```python
from build123d import *

# Parameters (mm, degrees)
SKETCH1_W           = 50
SKETCH1_H           = 200
BOSS_EXTRUDE1_DEPTH = 5.2
SKETCH2_W           = 4.9
SKETCH2_H           = 7.8
SKETCH2_W_2         = 5.7
SKETCH2_H_2         = 9
SKETCH2_W_3         = 25
SKETCH2_H_3         = 4.9
CUT_EXTRUDE1_DEPTH  = 5.2
CHAMFER2_SIZE       = 2.6


with BuildPart() as part:
    # Sketch1 → Boss-Extrude1 (new body)
    with BuildSketch(Plane(origin=(0, 0, 0), x_dir=(1, 0, 0), z_dir=(0, 1, 0))):
        with Locations((25, 100)):
            Rectangle(SKETCH1_W, SKETCH1_H)
    extrude(amount=BOSS_EXTRUDE1_DEPTH)

    # Sketch2 → Cut-Extrude1 (cut)
    with BuildSketch(Plane(origin=(0, 5.2, 0), x_dir=(1, 0, 0), z_dir=(0, 1, 0))):
        with Locations((12.45, 196.1)):
            Rectangle(SKETCH2_W, SKETCH2_H)
        with Locations((37.15, 195.5)):
            Rectangle(SKETCH2_W_2, SKETCH2_H_2)
        with Locations((37.5, 100)):
            Rectangle(SKETCH2_W_3, SKETCH2_H_3)
        with Locations((12.45, 3.9)):
            Rectangle(SKETCH2_W, SKETCH2_H)
        with Locations((37.15, 4.5)):
            Rectangle(SKETCH2_W_2, SKETCH2_H_2)
    extrude(amount=-CUT_EXTRUDE1_DEPTH, mode=Mode.SUBTRACT)

    # Chamfer2
    chamfer2_edges = [part.edges().sort_by_distance(p)[0] for p in [
        (10, 2.6, 0),
        (14.9, 2.6, 0),
        (34.3, 2.6, 0),
        (40, 2.6, 0),
        (50, 2.6, -102.45),
        (50, 2.6, -97.55),
        (34.3, 2.6, -200),
        (40, 2.6, -200),
        (10, 2.6, -200),
        (14.9, 2.6, -200),
    ]]
    chamfer(chamfer2_edges, length=CHAMFER2_SIZE)


solid = part.part
```
Here's how the part is built. I have some questions about the finished solid (model axes, mm). A direction names the side the tool comes from. Coordinates: 2 decimals unless noted, no trailing zeros. Return JSON: item names as keys, results as strings. Group by question number.
Item 1: Will these pins go through, and if not, where does the flat tip stop? P1, Ø1.5, axis at x = 12.5, y = 1.5, coming from the +Z side; P2, Ø2.5, axis at x = 36, y = 2.5, coming from the +Z side.
Item 2: On a 3-axis mill with a long thin cutter (end or side, diameter ignored), from which of +Z, -Z, +X, -X, +Y, -Y can I reach the whole of each face in a straight line? I mean faces 5 (the face through (0, 3, -99)), 6 (the face through (34.3, 3, -194)), 7 (the face through (12, 3, -7.8)), 8 (the face through (46, 3, -200)), 9 (the face through (25, 3, -100)). Say none if no direction works.
Item 3: We'd pull the mould along X, two halves only. Please class faces 1 (the face through (25, 3, 0)), 2 (the face through (50, 3, -152)), 3 (the face through (37, 3, -191)), 4 (the face through (14.9, 3, -5)): +X half, -X half, draft (parallel to the pull), parting line (faces both ways), or undercut.
Item 4: I need wall thicknesses on line 1 (Z direction, x = 27.5, y = 4.65); line 2 (Z direction, x = 13.5, y = 3.3); line 3 (X direction, y = 2.35, z = -8.5). Which ranges of each line are inside material? Lowest first, please. Write a range as from..to.
Calculated:
{
 "1": {"P1": "stops at z = -7.8", "P2": "stops at z = -9"},
 "2": {"face 5": "+Z, -Z, -X, +Y, -Y", "face 6": "-Z, +Y, -Y", "face 7": "+Z, +Y, -Y", "face 8": "-Z, +X, -X, +Y, -Y", "face 9": "+X, +Y, -Y"},
 "3": {"face 1": "draft", "face 2": "+X half", "face 3": "undercut", "face 4": "undercut"},
 "4": {"line 1": "z = -200..-102.45, -97.55..0", "line 2": "z = -192.2..-7.8", "line 3": "x = 0..34.3, 40..50"}
}
